Could you check a few things on this drawing? It's one solid part, dimensions in mm from its lowest x, y, z. A direction names the side the tool comes from. Give positions to 0.01 mm unless a question says otherwise; leave off trailing zeros. Order: outer loops, then holes, each group sorted by start corner. A loop starts at its lowest first (then second) coordinate and runs counter-clockwise, first axis right, second up.
(1) If we mould it in two halves opening along Y, with no side actions, what happens to the marked faces 4, 5 and 6? For each: released by +Y, released by -Y, zero draft, split by the parting line, or undercut.
(2) On a 3-axis mill with a long thin cutter (end or side, diameter ignored), from which of +Z, -Z, +X, -X, +Y, -Y can I reach the whole of each face in a straight line? I mean the marked faces 1, 2 and 3. Say none if no direction works.
(3) If I drill on probe 1 along Y at (x, z) = (19, 15.5) (1 decimal); probe 2 along X at (y, z) = (6.75, 18) (1 decimal); probe 3 along Y at (x, z) = (2, 11) (1 decimal), over which ranges is the centre line in solid material (lowest first)?
(4) Imagine slicing it at B-B, the plane z = 6.5. Write out the boundary of the cut face in (x, y) (1 decimal), then the cut area to 3 significant figures.
(5) Imagine slicing it at D-D, the plane z = 21. Write out the boundary of the cut face in (x, y) (1 decimal), then the cut area to 3 significant figures.
(6) Imagine slicing it at A-A, the plane x = 5. Write out the boundary of the cut face in (y, z) (1 decimal).
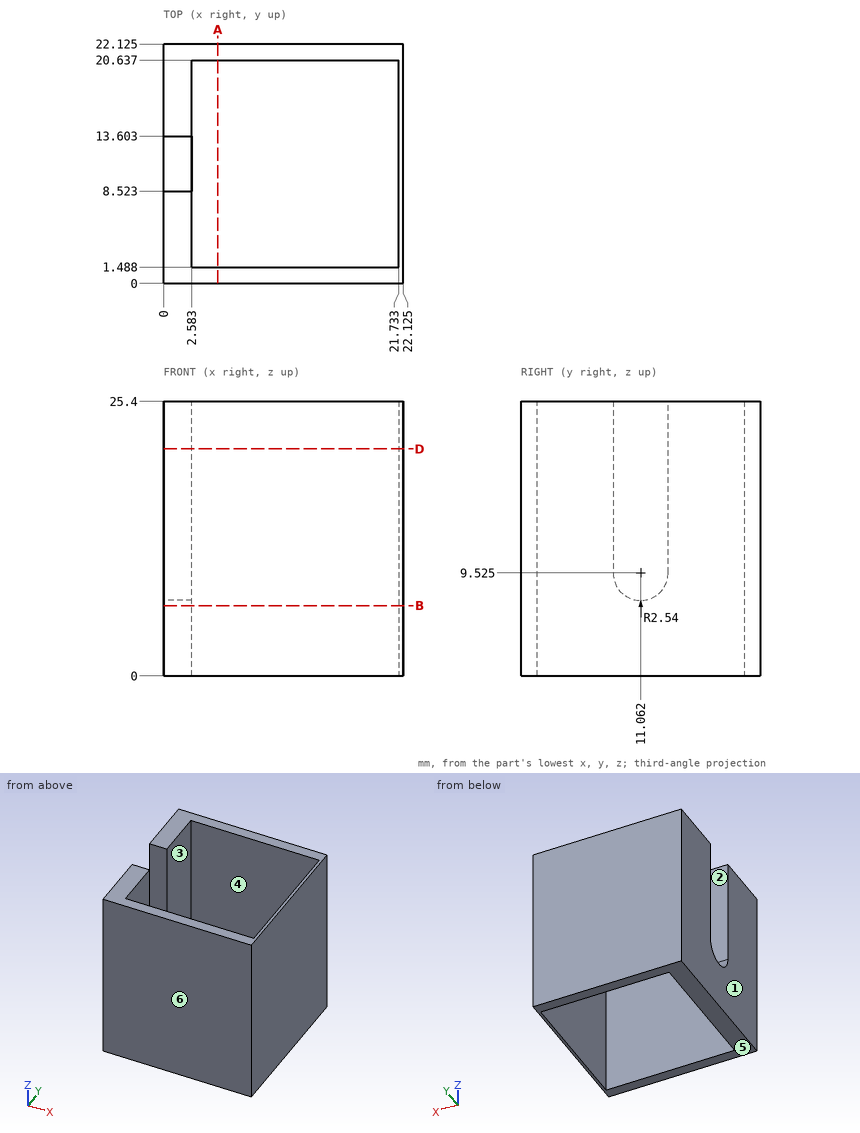
Answer block:
1. face 4: undercut
1. face 5: zero draft
1. face 6: released by -Y
2. face 1: +Z, -Z, -X, +Y, -Y
2. face 2: +Z, -X
2. face 3: +Z, -Z
3. probe 1: y = 0 to 1.5, 20.6 to 22.1
3. probe 2: x = 0 to 2.6, 21.7 to 22.1
3. probe 3: y = 0 to 8.5, 13.6 to 22.1
4. outline: (0, 0) - (22.1, 0) - (22.1, 22.1) - (0, 22.1) - close; hole (2.6, 1.5) - (21.7, 1.5) - (21.7, 20.6) - (2.6, 20.6) - close
4. area: 123 mm2
5. outline: (0, 0) - (22.1, 0) - (22.1, 22.1) - (0, 22.1) - (0, 13.6) - (2.6, 13.6) - (2.6, 20.6) - (21.7, 20.6) - (21.7, 1.5) - (2.6, 1.5) - (2.6, 8.5) - (0, 8.5) - close
5. area: 110 mm2
6. outline: (0, 0) - (1.5, 0) - (1.5, 25.4) - (0, 25.4) - close; (20.6, 0) - (22.1, 0) - (22.1, 25.4) - (20.6, 25.4) - close
